from build123d import *

# Parameters (mm, degrees)
F0_R     = 25.4
F1_DEPTH = 5.08
F3_DEPTH = 25.4
F4_R     = 2.54
F5_R     = 2.54
F6_DEPTH = 25.4
F8_DEPTH = 5.08


with BuildPart() as f1:
    # F0 (on Top) → F1 (new body)
    with BuildSketch(Plane.XY):
        Circle(F0_R)
    extrude(amount=F1_DEPTH)

    # F2 (on face) → F3 (cut)
    with BuildSketch(Plane.XY.offset(5.08)):
        with BuildLine():
            ThreePointArc((-6.6100981471, -22.7330046286), (-9.5231262698, -15.6860792516), (-6.3329048366, -8.7602307605))
            ThreePointArc((-6.3329048366, -8.7602307605), (-6.3640275163, -8.6837329224), (-6.3955051853, -8.6073804713))
            Line((-6.3955051853, -8.6073804713), (-6.4190231614, -8.5806554984))
            ThreePointArc((-6.4190231614, -8.5806554984), (-18.6783561202, -10.4151947963), (-25.4, -3e-09))
            ThreePointArc((-25.4, -3e-09), (-20.4128361311, -15.1154265929), (-7.4097542481, -24.295175282))
            ThreePointArc((-7.4097542481, -24.295175282), (-6.9906405345, -23.523962051), (-6.6100981471, -22.7330046286))
        make_face()
        with BuildLine():
            Line((-13.97, 0), (-6.4190231614, -8.5806554984))
            ThreePointArc((-6.4190231614, -8.5806554984), (-6.4144876205, -8.5766620945), (-6.4099541915, -8.5726662931))
            ThreePointArc((-6.4099541915, -8.5726662931), (-9.482325957, -3.6622711754), (-13.97, 0))
        make_face()
        with BuildLine():
            ThreePointArc((-25.4, -3e-09), (-18.6783561202, -10.4151947963), (-6.4190231614, -8.5806554984))
            Line((-6.4190231614, -8.5806554984), (-13.97, 0))
            ThreePointArc((-13.97, 0), (-19.3966889497, 2.0254618044), (-25.1864455812, 2.1991472264))
            ThreePointArc((-25.1864455812, 2.1991472264), (-25.3464861227, 1.1047458984), (-25.4, -3e-09))
        make_face()
        with BuildLine():
            ThreePointArc((-5.0375846352, -15.4223424331), (-5.3644186356, -12.0289080974), (-6.3329048366, -8.7602307605))
            ThreePointArc((-6.3329048366, -8.7602307605), (-9.5231262698, -15.6860792516), (-6.6100981471, -22.7330046286))
            ThreePointArc((-6.6100981471, -22.7330046286), (-5.4351580244, -19.1612787953), (-5.0375846352, -15.4223424331))
        make_face()
        with BuildLine():
            ThreePointArc((-7.4097542481, -24.295175282), (-3.7458341923, -25.1222754981), (3.3e-08, -25.4))
            ThreePointArc((3.3e-08, -25.4), (-3.3627869226, -24.7866378468), (-6.2924806988, -23.0255462487))
            Line((-6.2924806988, -23.0255462487), (-7.4097542481, -24.295175282))
        make_face()
        with BuildLine():
            Line((7.4097542481, -24.295175282), (6.2924806988, -23.0255462487))
            ThreePointArc((6.2924806988, -23.0255462487), (3.3627869535, -24.7866378352), (3.3e-08, -25.4))
            ThreePointArc((3.3e-08, -25.4), (3.745834225, -25.1222754933), (7.4097542481, -24.295175282))
        make_face()
        with BuildLine():
            ThreePointArc((6.3329048366, -8.7602307605), (8.690412636, -11.9759804802), (9.525, -15.875))
            ThreePointArc((9.525, -15.875), (8.7660370137, -19.6008851398), (6.6100981471, -22.7330046286))
            ThreePointArc((6.6100981471, -22.7330046286), (6.9906405345, -23.523962051), (7.4097542481, -24.295175282))
            ThreePointArc((7.4097542481, -24.295175282), (20.412836132, -15.1154265917), (25.4, 0))
            ThreePointArc((25.4, 0), (18.6783561215, -10.4151947957), (6.4190231614, -8.5806554984))
            Line((6.4190231614, -8.5806554984), (6.3955051853, -8.6073804713))
            ThreePointArc((6.3955051853, -8.6073804713), (6.3640275163, -8.6837329224), (6.3329048366, -8.7602307605))
        make_face()
        with BuildLine():
            Line((13.97, 0), (6.4190231614, -8.5806554984))
            ThreePointArc((6.4190231614, -8.5806554984), (18.6783561215, -10.4151947957), (25.4, 0))
            ThreePointArc((25.4, 0), (25.3464861226, 1.1047458999), (25.1864455812, 2.1991472264))
            ThreePointArc((25.1864455812, 2.1991472264), (19.3966889497, 2.0254618044), (13.97, 0))
        make_face()
        with BuildLine():
            ThreePointArc((6.6100981471, -22.7330046286), (8.7660370137, -19.6008851398), (9.525, -15.875))
            ThreePointArc((9.525, -15.875), (8.690412636, -11.9759804802), (6.3329048366, -8.7602307605))
            ThreePointArc((6.3329048366, -8.7602307605), (5.0410822649, -15.7749944968), (6.6100981471, -22.7330046286))
        make_face()
        with BuildLine():
            ThreePointArc((6.4099541915, -8.5726662931), (6.4144876205, -8.5766620945), (6.4190231614, -8.5806554984))
            Line((6.4190231614, -8.5806554984), (13.97, 0))
            ThreePointArc((13.97, 0), (9.482325957, -3.6622711754), (6.4099541915, -8.5726662931))
        make_face()
        with BuildLine():
            Line((-7.4097542481, -24.295175282), (-6.2924806988, -23.0255462487))
            ThreePointArc((-6.2924806988, -23.0255462487), (-6.4529474172, -22.8810755514), (-6.6100981471, -22.7330046286))
            ThreePointArc((-6.6100981471, -22.7330046286), (-6.9906405345, -23.523962051), (-7.4097542481, -24.295175282))
        make_face()
        with BuildLine():
            ThreePointArc((7.4097542481, -24.295175282), (6.9906405345, -23.523962051), (6.6100981471, -22.7330046286))
            ThreePointArc((6.6100981471, -22.7330046286), (6.4529474172, -22.8810755514), (6.2924806988, -23.0255462487))
            Line((6.2924806988, -23.0255462487), (7.4097542481, -24.295175282))
        make_face()
        with BuildLine():
            ThreePointArc((-25.1864455812, 2.1991472264), (-25.2462602872, 2.1910029214), (-25.306046997, 2.1826555809))
            ThreePointArc((-25.306046997, 2.1826555809), (-25.3765008791, 1.0923383792), (-25.4, -3e-09))
            ThreePointArc((-25.4, -3e-09), (-25.3464861227, 1.1047458984), (-25.1864455812, 2.1991472264))
        make_face()
        with BuildLine():
            ThreePointArc((25.1864455812, 2.1991472264), (25.3464861226, 1.1047458999), (25.4, 0))
            ThreePointArc((25.4, 0), (25.376500879, 1.0923383807), (25.306046997, 2.1826555809))
            ThreePointArc((25.306046997, 2.1826555809), (25.2462602872, 2.1910029214), (25.1864455812, 2.1991472264))
        make_face()
    extrude(amount=-F3_DEPTH, mode=Mode.SUBTRACT)

    # F4
    f4_edges = [f1.edges().sort_by_distance(p)[0] for p in [
        (-25.306047, 2.182656, 2.54),
        (-6.610098, -22.733005, 2.54),
        (6.610098, -22.733005, 2.54),
        (25.306047, 2.182656, 2.54),
    ]]
    fillet(f4_edges, radius=F4_R)

    # F5 (on face) → F6 (cut)
    with BuildSketch(Plane.XY.offset(5.08)):
        Circle(F5_R)
    extrude(amount=-F6_DEPTH, mode=Mode.SUBTRACT)

    # F7 (on face) → F8 (join)
    with BuildSketch(Plane.XY.offset(5.08)):
        with BuildLine():
            ThreePointArc((0, -13.335), (-1.7960512242, -17.6710512242), (2.54, -15.875))
            ThreePointArc((2.54, -15.875), (1.7960512242, -14.0789487758), (0, -13.335))
        make_face()
    extrude(amount=F8_DEPTH)


solid = f1.part
Input: part model. Units: mm. Frame: model coordinates. Coordinates: 2 decimals unless noted, no trailing zeros. Loops run counter-clockwise (first coordinate to the right, second up) from the corner with the lowest first, then second, coordinate; pieces in that order, holes last. Notation, with made-up numbers: (9, 63) -> (58, 63) arc R15 cw to (58, 72) -> close; hole circle Ø4 at (22.25, -13.75). An arc over 180 degrees is marked (long way). One line per item, written item: value.
(1) Cut plane B-B (y = -20). Output: boundary loops of the cut face in (x, z), then the cut area to 3 significant figures.
Answer below:
outline: (-5.64, 0) -> (5.64, 0) -> (5.64, 5.08) -> (-5.64, 5.08) -> close
area: 57.3 mm2
(2) Cut plane A-A (z = 9.5). Output: boundary loops of the cut face in (x, y) (3 decimals).
Answer below:
outline: circle Ø5.08 at (0, -15.875)
(3) Pin query (flat end, axial travel): pin 1 Ø6 at (x, z) = (-4, 1.5) entering from +Y; pin 2 Ø6 at (y, z) = (-14.5, 7.5) entering from -X; pin 3 Ø5 at (x, z) = (5, 2.5) entering from +Y. Return the tip coordinate at first contact, or that it passes through.
Answer below:
pin 1: stops at y = 25.38
pin 2: stops at x = -5.24
pin 3: stops at y = 25.28
(4) Draft query along Y for faces 1 (the face through (0, 6, 0)), 2 (the face through (0.482, 25.395, 2.504)), 3 (the face through (-0.33, 2.52, 2.58)). Return one class per face: pulls with the +Y half, pulls with the -Y half, needs draft (parallel to the pull), parting line crosses it, or undercut.
Answer below:
face 1: needs draft
face 2: pulls with the +Y half
face 3: undercut
(5) Ray query, line 1 along Z through (x, y) = (-3.5, -3); line 2 along X through (y, z) = (-15.5, 2.75); line 3 along X through (y, z) = (17, 2.75). Return the intervals inside material, ascending.
Answer below:
line 1: z = 0 to 5.08
line 2: x = -5.04 to 5.04
line 3: x = -18.87 to 18.87
(6) Cut plane C-C (x = 16). Output: boundary loops of the cut face in (y, z).
Answer below:
outline: (1, 0) -> (19.73, 0) -> (19.73, 5.08) -> (1, 5.08) -> close
